Here's how the part is built. I have some questions about the finished solid (model axes, mm). A direction names the side the tool comes from. Coordinates: 2 decimals unless noted, no trailing zeros. Write each loop counter-clockwise with the first axis right and the second up, starting at its lowest first coordinate (ties: lowest second). Pieces come first, ordered by that corner, then holes.
Item 1: If I drill on line 1 (Z direction, x = 0, y = 20.5); line 2 (Z direction, x = -4, y = 30), over which ranges is the centre line in solid material (lowest first)?
Item 2: If we section it at C-C (x = 0): Please give me the cut outline in (y, z), then the cut area to 3 significant figures.
Item 3: I'm going to push flat-ended pins straight in: pin 1 Ø2.5 at (x, y) = (-8, 20) entering from +Z; pin 2 Ø3.5 at (x, y) = (-8, 18) entering from -Z; pin 3 Ø2 at (x, z) = (0.5, 13) entering from +Y. Where does each tip first touch, or does it pass through?
Item 4: For faces 1 (the face through (0, 34, -8.2)), 2 (the face through (-8, 14, 0)), 3 (the face through (1.2, 9, 12.1)), which set-ups out of +Z, -Z, +X, -X, +Y, -Y let a thin tool reach every point of the face, with its end or its side?
Item 5: If we section it at D-D (y = 12.5): Please give me the cut outline in (x, z).
Item 6: We'd pull the mould along X, two halves only. Please class faces 4 (the face through (8, 24, 0)), 5 (the face through (9.237, 22.339, -3.83)), 6 (the face through (0, 9, 0)): +X half, -X half, draft (parallel to the pull), parting line (faces both ways), or undercut.
Item 7: If we section it at A-A (z = 0): Please give me the cut outline in (x, y).
Item 8: If we section it at B-B (y = 19.5): Please give me the cut outline in (x, z).
Autodesk Inventor part; units mm, degrees
ref_plane "YZ Plane" through (0, 0, 0) normal (1, 0, 0) x (0, 1, 0)
ref_plane "XZ Plane" through (0, 0, 0) normal (0, 1, 0) x (-1, 0, 0)
ref_plane "XY Plane" through (0, 0, 0) normal (0, 0, 1) x (1, 0, 0)
sketch "Sketch1" plane through (0, 0, 0) normal (0, 1, 0) x (-1, 0, 0)
  circle A0 centre (0, 0) radius 20
  dimension "d0" = 40
extrude "Extrusion1" add sketch "Sketch1" along normal blind 9 draft -30
sketch "Sketch2" plane through (0, 9, 0) normal (0, 1, 0) x (1, 0, 0)
  circle A0 centre (0, 0) radius 10
  dimension "d3" = 20
extrude "Extrusion2" add sketch "Sketch2" along normal blind 25
sketch "Sketch3" plane through (0, 34, 0) normal (0, 1, 0) x (1, 0, 0)
  circle A0 centre (0, 0) radius 7
  dimension "d6" = 14
extrude "Extrusion3" cut sketch "Sketch3" against normal up to surface (25 mm away)
sketch "Sketch4" plane through (0, 0, 0) normal (1, 0, 0) x (0, 1, 0)
  line L0 (24, -3) -> (14, -3)
  line L1 (14, -3) -> (14, 3)
  line L2 (14, 3) -> (24, 3)
  line L3 (24, 3) -> (24, -3)
  line L4 (9, 7) -> (9, -7)
  point P0 (0, 0)
  dimension "d9" = 10
  dimension "d10" = 6
  dimension "d11" = 3
  dimension "d12" = 5
extrude "Extrusion4" cut sketch "Sketch4" along normal through all both and the other way through all
fillet "Fillet1" radius 2 1 edges at (-10, 9, 0)
chamfer "Chamfer1" distance 1 angle 45 1 edges at (-7, 34, 0)
properties part number "Foot Stamp"
Answer list:
1. line 1: z = -10 to -7, 7 to 10
1. line 2: z = -9.17 to -5.74, 5.74 to 9.17
2. outline: (0, -20) - (9, -14.8) - (9, -12) arc R2 cw to (11, -10) - (34, -10) - (34, -8) - (33, -7) - (9, -7) - (9, 7) - (33, 7) - (34, 8) - (34, 10) - (11, 10) arc R2 cw to (9, 12) - (9, 14.8) - (0, 20) - close
2. area: 464 mm2
3. pin 1: stops at z = 7.38
3. pin 2: stops at z = -7.81
3. pin 3: stops at y = 9
4. face 1: +Z, -Z, +X, -X, +Y
4. face 2: +X, -X
4. face 3: +Y
5. outline: circle Ø20 at (0, 0); hole circle Ø14 at (0, 0)
6. face 4: draft
6. face 5: parting line
6. face 6: undercut
7. outline: (-20, 0) - (20, 0) - (14.8, 9) - (12, 9) arc R2 cw to (10, 11) - (10, 14) - (7, 14) - (7, 9) - (-7, 9) - (-7, 14) - (-10, 14) - (-10, 11) arc R2 cw to (-12, 9) - (-14.8, 9) - close; (-10, 24) - (-7, 24) - (-7, 33) - (-8, 34) - (-10, 34) - close; (7, 24) - (10, 24) - (10, 34) - (8, 34) - (7, 33) - close
8. outline: (-9.54, -3) arc R10 ccw to (9.54, -3) - (6.32, -3) arc R7 cw to (-6.32, -3) - close; (-9.54, 3) - (-6.32, 3) arc R7 cw to (6.32, 3) - (9.54, 3) arc R10 ccw to start
